Geometry: final body of the model. Coordinates: model frame, mm. A direction names the side the tool comes from. Coordinates: 2 decimals unless noted, no trailing zeros. Loops run counter-clockwise (first coordinate to the right, second up) from the corner with the lowest first, then second, coordinate; pieces in that order, holes last. Notation, with made-up numbers: (-8, 67) -> (44, 67) arc R13 ccw to (44, 75) -> close; hole circle Ø11 at (-12, 37.25). An arc over 180 degrees is marked (long way). One line per item, written item: value. Start each with the question number.
Item 1: Mould query, pull axis X, two halves, no side actions, for faces 4 (the cylindrical face through (4.859, 4.521, -0.267)), 5 (the cylindrical face through (-1.48, 10.05, 14.25)), 6 (the flat face through (-7.8, 14, -12)), 7 (the flat face through (22.7, 5, -25)). Classes: +X half, -X half, draft (parallel to the pull), parting line (faces both ways), or undercut.
Item 2: Ray query, probe 1 along Z at (x, y) = (6.2, 1.1); probe 2 along X at (y, z) = (0.7, -23.5); probe 3 along X at (y, z) = (1.3, -3.5). Return the intervals inside material, ascending. Write a range as from..to.
Item 3: Section query C-C on z = -12.2. Return loops of the section in (x, y).
Item 4: Contact query for flat-ended pins moving along their axis: pin 1 Ø2.5 at (x, z) = (6.2, -23.5) entering from +Y; pin 2 Ø10 at (x, y) = (24.5, 18.5) entering from -Z; pin 3 Ø2.5 at (y, z) = (4.5, -24.5) entering from -X; pin 4 Ø10 at (y, z) = (7, 6.5) entering from -X. Output: stop coordinate, or through.
Item 5: Section query A-A on x = 0.7. Return loops of the section in (y, z).
Item 6: Section query B-B on x = 6.2. Give the number of separate pieces and of enclosed holes in the cut face, then the cut area to 3 significant figures.
Item 7: Section query D-D on y = 19. Return loops of the section in (x, z).
Item 8: Set-up query: faces 1 (the flat face through (6.93, 3, -25.1)), 2 (the flat face through (11, 14, -8.7)), 3 (the flat face through (28, 8, 1.5)). Return all of +Z, -Z, +X, -X, +Y, -Y with unobstructed straight access to the full face (end or side cutting, diameter ignored); none if empty.
from build123d import *

# Parameters (mm, degrees)
SKETCH_1_R          = 1.6
EXTRUDE_1_DEPTH     = 6
SKETCH_2_R          = 3.5
CUT_EXTRUDE_1_DEPTH = 3
SKETCH_3_W          = 48
SKETCH_3_H          = 7
EXTRUDE_2_DEPTH     = 16
SKETCH_5_R          = 2.75
CUT_EXTRUDE_2_DEPTH = 7
SKETCH_6_R          = 1.6
EXTRUDE_3_DEPTH     = 5
SKETCH_7_R          = 1.75
EXTRUDE_4_DEPTH     = 3
CHAMFER_1_SIZE      = 10
CUT_EXTRUDE_START   = -11
SKETCH_8_R          = 1.6
CUT_EXTRUDE_3_DEPTH = 11
SKETCH_9_R          = 1.75
CUT_EXTRUDE_4_DEPTH = 7


with BuildPart() as part:
    # Эскиз1 → Бобышка-Вытянуть1 (new body)
    with BuildSketch(Plane(origin=(0, 0, 0), x_dir=(1, 0, 0), z_dir=(0, 1, 0))):
        Polygon((0, 0), (0, 27), (32.4, 27), (32.4, 0), (35.4, 0), (35.4, -9), (-3, -9), (-3, 0), align=None)
        with Locations(Location((6.2, 23.5, 0), (0, 0, 270))):
            Circle(SKETCH_1_R, mode=Mode.SUBTRACT)
        with Locations(Location((26.2, 23.5, 0), (0, 0, 270))):
            Circle(SKETCH_1_R, mode=Mode.SUBTRACT)
        with Locations(Location((6.2, 3.5, 0), (0, 0, 270))):
            Circle(SKETCH_1_R, mode=Mode.SUBTRACT)
        with Locations(Location((26.2, 3.5, 0), (0, 0, 270))):
            Circle(SKETCH_1_R, mode=Mode.SUBTRACT)
        with Locations(Location((31.7, -4.5, 0), (0, 0, 270))):
            Circle(SKETCH_1_R, mode=Mode.SUBTRACT)
        with Locations(Location((0.7, -4.5, 0), (0, 0, 270))):
            Circle(SKETCH_1_R, mode=Mode.SUBTRACT)
    extrude(amount=EXTRUDE_1_DEPTH)

    # Эскиз2 → Вырез-Вытянуть1 (cut)
    with BuildSketch(Plane(origin=(0, 6, 0), x_dir=(1, 0, 0), z_dir=(0, 1, 0))):
        with Locations(Location((26.2, 3.5, 0), (0, 0, 270))):
            Circle(SKETCH_2_R)
        with Locations(Location((6.2, 3.5, 0), (0, 0, 270))):
            Circle(SKETCH_2_R)
        with BuildLine():
            Line((29.7, 23.5), (29.7, 27))
            Line((29.7, 27), (22.7, 27))
            Line((22.7, 27), (22.7, 23.5))
            ThreePointArc((22.7, 23.5), (26.2, 20), (29.7, 23.5))
        make_face()
        with BuildLine():
            Line((9.7, 23.5), (9.7, 27))
            Line((9.7, 27), (2.7, 27))
            Line((2.7, 27), (2.7, 23.5))
            ThreePointArc((2.7, 23.5), (6.2, 20), (9.7, 23.5))
        make_face()
    extrude(amount=-CUT_EXTRUDE_1_DEPTH, mode=Mode.SUBTRACT)

    # Эскиз3 → Бобышка-Вытянуть2 (add)
    with BuildSketch(Plane(origin=(0, 6, 0), x_dir=(1, 0, 0), z_dir=(0, 1, 0))):
        with Locations((16.2, 12.2)):
            Rectangle(SKETCH_3_W, SKETCH_3_H)
    extrude(amount=EXTRUDE_2_DEPTH)

    # Эскиз5 → Вырез-Вытянуть2 (cut)
    with BuildSketch(Plane(origin=(0, 0, -15.7), x_dir=(-1, 0, 0), z_dir=(0, 0, -1))):
        with Locations((-35.25, 14)):
            Circle(SKETCH_5_R)
        with Locations((2.85, 14)):
            Circle(SKETCH_5_R)
    extrude(amount=-CUT_EXTRUDE_2_DEPTH, mode=Mode.SUBTRACT)

    # Эскиз6 → Бобышка-Вытянуть3 (add)
    with BuildSketch(Plane(origin=(0, 6, 0), x_dir=(1, 0, 0), z_dir=(0, 1, 0))):
        Polygon((35.4, -7.5), (-3, -7.5), (-3, -1.5), (12.2, -1.5), (12.2, 8.7), (20.2, 8.7), (20.2, -1.5), (35.4, -1.5), align=None)
        with Locations(Location((31.7, -4.5, 0), (0, 0, 270))):
            Circle(SKETCH_6_R, mode=Mode.SUBTRACT)
        with Locations(Location((0.7, -4.5, 0), (0, 0, 270))):
            Circle(SKETCH_6_R, mode=Mode.SUBTRACT)
    extrude(amount=EXTRUDE_3_DEPTH)

    # Эскиз7 → Бобышка-Вытянуть4 (add)
    with BuildSketch(Plane.ZY):
        Polygon((7.5, 12.97640534), (18.99998535, 12.97640534), (18.99998535, 6), (9, 6), (9, 0), (-6, 0), (-6, 12.97640534), (1.5, 12.97640534), (1.5, 11), (7.5, 11), align=None)
        with Locations((-3, 10)):
            Circle(SKETCH_7_R, mode=Mode.SUBTRACT)
        with Locations((15.99998535, 9.97640534)):
            Circle(SKETCH_7_R, mode=Mode.SUBTRACT)
    extrude(amount=EXTRUDE_4_DEPTH)

    # Фаска1
    chamfer_1_edges = [part.edges().sort_by_distance(p)[0] for p in [
        (16.2, 11, -8.7),
    ]]
    chamfer(chamfer_1_edges, length=CHAMFER_1_SIZE)

    # Эскиз8 → Вырез-Вытянуть3 (cut)
    with BuildSketch(Plane(origin=(0, 11, 0), x_dir=(1, 0, 0), z_dir=(0, 1, 0)).offset(CUT_EXTRUDE_START)):
        with Locations(Location((0.7, -4.5, 0), (0, 0, 270))):
            Circle(SKETCH_8_R)
    extrude(amount=CUT_EXTRUDE_3_DEPTH, mode=Mode.SUBTRACT)

    # Эскиз9 → Вырез-Вытянуть4 (cut)
    with BuildSketch(Plane(origin=(0, 22, 0), x_dir=(1, 0, 0), z_dir=(0, 1, 0))):
        with Locations(Location((26.2, 12.2, 0), (0, 0, 270))):
            Circle(SKETCH_9_R)
        with Locations(Location((6.2, 12.2, 0), (0, 0, 270))):
            Circle(SKETCH_9_R)
    extrude(amount=-CUT_EXTRUDE_4_DEPTH, mode=Mode.SUBTRACT)


solid = part.part
Reply:
1. face 4: undercut
1. face 5: draft
1. face 6: -X half
1. face 7: undercut
2. probe 1: z = -27..-25.1, -21.9..-5.1, -1.9..9
2. probe 2: x = 0..4.6, 7.8..24.6, 27.8..32.4
2. probe 3: x = -3..4.6, 7.8..24.6, 27.8..32.4
3. outline: (-7.8, 6) -> (0, 6) -> (0, 0) -> (32.4, 0) -> (32.4, 6) -> (40.2, 6) -> (40.2, 22) -> (27.95, 22) -> (27.95, 15) -> (24.45, 15) -> (24.45, 22) -> (7.95, 22) -> (7.95, 15) -> (4.45, 15) -> (4.45, 22) -> (-7.8, 22) -> close; hole circle Ø5.5 at (-2.85, 14); hole circle Ø5.5 at (35.25, 14)
4. pin 1: passes through
4. pin 2: stops at z = -15.7
4. pin 3: stops at x = 0
4. pin 4: stops at x = -3
5. outline: (0, -27) -> (6, -27) -> (6, -15.7) -> (22, -15.7) -> (22, -8.7) -> (6, -8.7) -> (6, 1.5) -> (11, 1.5) -> (11, 2.9) -> (0, 2.9) -> close; (0, 6.1) -> (11, 6.1) -> (11, 7.5) -> (6, 7.5) -> (6, 9) -> (0, 9) -> close
6. separate pieces: 3
6. enclosed holes: 0
6. area: 272 mm²
7. outline: (-7.8, -15.7) -> (40.2, -15.7) -> (40.2, -8.7) -> (20.2, -8.7) -> (20.2, -6.7) -> (12.2, -6.7) -> (12.2, -8.7) -> (-7.8, -8.7) -> close; hole circle Ø3.5 at (6.2, -12.2); hole circle Ø3.5 at (26.2, -12.2)
8. face 1: -Z, +Y
8. face 2: +Y
8. face 3: +X, +Y
